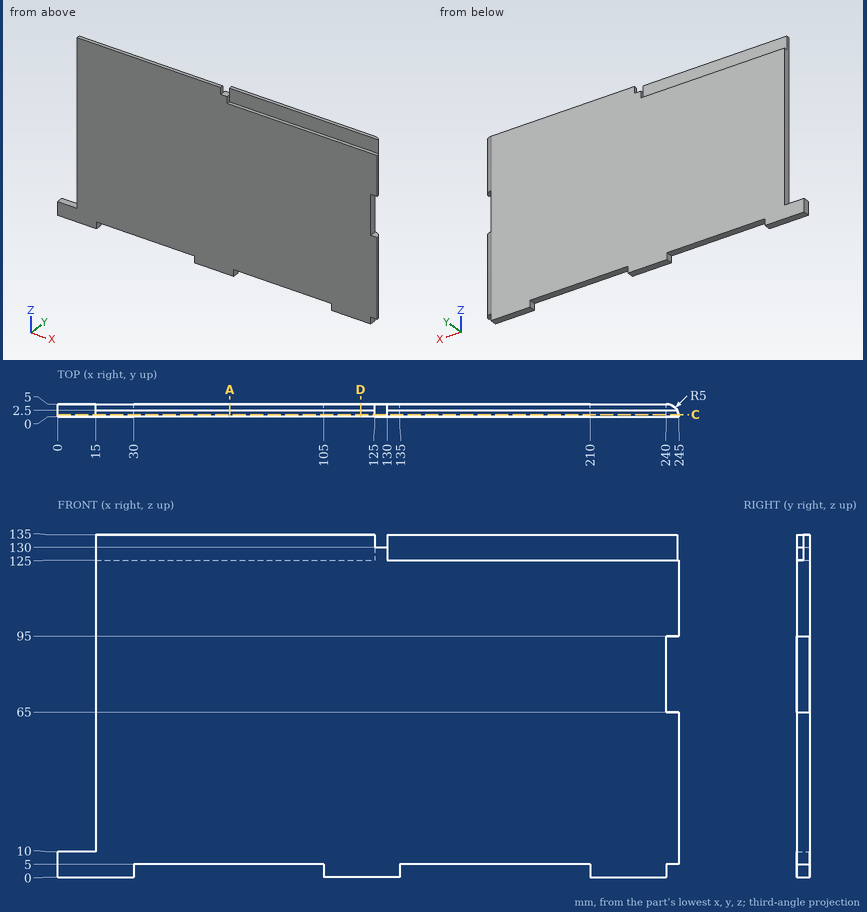
Study the drawing (mm; zero at the part's minimum x, y, z) and answer. Give positions to 0.01 mm unless a question says otherwise; leave off trailing zeros. Order: outer loops, then holes, each group sorted by start corner. A loop starts at its lowest first (then second) coordinate and runs counter-clockwise, first axis right, second up. Notation, with made-up numbers: M 59.25,62.25 L 118.25,62.25 A33 ccw 118.25,98.25 Z; hole C -0.5,45 d8. An arc over 180 degrees is marked long. Put each result on its own line as item: value. Start each with the question number.
Item 1: The part is cut by section D-D, the plane x = 119.5. Determine the outline of the cut face in (y, z), and give its area (3 significant figures).
Item 2: The part is cut by section C-C, the plane y = 0.85. Determine the outline of the cut face in (x, z).
Item 3: The part is cut by section A-A, the plane x = 68. Determine the outline of the cut face in (y, z), and give its area (3 significant figures).
Item 4: Flat-ended cylindrical pins translate along their axes: P1, Ø1, axis at x = 47, y = 4.5, coming from the -Z side; P2, Ø8, axis at x = 86, z = 129.5, coming from the +Y side; P3, Ø2.5, axis at y = 1.5, z = 3.5, coming from the +X side. Find the tip coordinate at first contact, or state that the pin passes through.
Item 5: Find the intervals of material crossed by line 1 along Z through (x, y) = (103, 3.65); line 2 along Z through (x, y) = (180.5, 2.7); line 3 along X through (y, z) = (0.65, 83), in increasing order.
Answer key:
1. outline: M 0,0 L 5,0 L 5,125 L 2.5,125 L 2.5,135 L 0,135 Z
1. area: 650 mm²
2. outline: M 0,0 L 30,0 L 30,5 L 105,5 L 105,0 L 135,0 L 135,5 L 210,5 L 210,0 L 240,0 L 240,5 L 244.93,5 L 244.93,65 L 240,65 L 240,95 L 244.93,95 L 244.93,125 L 130,125 L 130,130 L 125,130 L 125,135 L 15,135 L 15,10 L 0,10 Z
3. outline: M 0,5 L 5,5 L 5,125 L 2.5,125 L 2.5,135 L 0,135 Z
3. area: 625 mm²
4. P1: stops at z = 5
4. P2: stops at y = 2.5
4. P3: stops at x = 240
5. line 1: z = 5 to 125
5. line 2: z = 5 to 135
5. line 3: x = 15 to 240
